Autodesk Inventor part; units mm, degrees
ref_plane "YZ Plane" through (0, 0, 0) normal (1, 0, 0) x (0, 1, 0)
ref_plane "XZ Plane" through (0, 0, 0) normal (0, 1, 0) x (-1, 0, 0)
ref_plane "XY Plane" through (0, 0, 0) normal (0, 0, 1) x (1, 0, 0)
sketch "Sketch1" plane through (0, 0, 0) normal (0, 1, 0) x (-1, 0, 0)
  line L0 (40.1367, 46.4954) -> (-10.6633, 46.4954)
  line L1 (-10.6633, 46.4954) -> (-10.6633, -55.1046)
  line L2 (-10.6633, -55.1046) -> (40.1367, -55.1046)
  line L3 (40.1367, -55.1046) -> (40.1367, 46.4954)
  circle A0 centre (14.7367, -4.3046) radius 12.7
  point P0 (0, 0)
  dimension "d0" = 101.6
  dimension "d1" = 50.8
  dimension "d21" = 25.4
  dimension "d22" = 50.8
extrude "Extrusion1" add sketch "Sketch1" along normal blind 25.4
sketch "Sketch2" plane through (-40.1367, 0, 46.4954) normal (0, 0, 1) x (1, 0, 0)
  line L0 (12.7, 19.8094) -> (36.1, 19.8094)
  line L1 (38.1, 17.8094) -> (38.1, 7.1094)
  line L2 (38.1, 7.1094) -> (12.7, 7.1094)
  line L3 (12.7, 7.1094) -> (12.7, 19.8094)
  line L4 (50.8, 0) -> (50.8, 25.4)
  line L5 (0, 0) -> (0, 25.4)
  arc A0 (38.1, 17.8094) -> (36.1, 19.8094) centre (36.1, 17.8094) ccw
  point P0 (40.1367, 0)
  point P1 (38.1, 19.8094)
  dimension "d5" = 25.4
  dimension "d6" = 12.7
  dimension "d7" = 12.7
  dimension "d8" = 12.7
  dimension "d9" = 12.7
  dimension "d10" = 2
extrude "Extrusion2" cut sketch "Sketch2" against normal up to next
equation "\"d1\" = 0.5 * d0"
equation "\"d21\" = 0.5 * d1"
equation "\"d22\" = 0.5 * d0"
properties part number "Block"
Geometry check sheet. Reference: the model listing, model coordinates, mm. A direction names the side the tool comes from. Give positions to 0.01 mm unless a question says otherwise; leave off trailing zeros. Order: outer loops, then holes, each group sorted by start corner. A loop starts at its lowest first (then second) coordinate and runs counter-clockwise, first axis right, second up.
1. Sectioned sample at C-C (x = -23.5). Record the boundary of the cut face in (y, z).
Completed:
outline: (0, -55.1) - (25.4, -55.1) - (25.4, -13.5) - (0, -13.5) - close; (0, 4.89) - (7.11, 4.89) - (7.11, 46.5) - (0, 46.5) - close; (19.81, 4.89) - (25.4, 4.89) - (25.4, 46.5) - (19.81, 46.5) - close
2. Depth check by flat-ended pin: pin 1 (1 mm diameter, centred on x = -15, z = -14.5, fed in from +Y); pin 2 (2 mm diameter, centred on x = -14.5, y = 12.5, fed in from +Z). Enter the tip coordinate at first touch or a pass-through.
Completed:
pin 1: passes through
pin 2: stops at z = -16.94
3. Sectioned sample at D-D (z = -7.5). Record the boundary of the cut face in (x, y).
Completed:
outline: (-40.14, 0) - (-27.03, 0) - (-27.03, 25.4) - (-40.14, 25.4) - close; (-2.45, 0) - (10.66, 0) - (10.66, 25.4) - (-2.45, 25.4) - close
4. Draft check along Z on faces 1 (the face through (-14, 13, -55.105)), 2 (the face through (-15.1, 6.9, 46.495)), 3 (the face through (-13.1, 12.5, -16.9)), 4 (the face through (-9, 25.4, 8)). Enter one of: pulls with the +Z half, pulls with the -Z half, needs draft (parallel to the pull), parting line crosses it, or undercut.
Completed:
face 1: pulls with the -Z half
face 2: pulls with the +Z half
face 3: undercut
face 4: needs draft
5. Sectioned sample at B-B (y = 9.5). Record the boundary of the cut face in (x, z).
Completed:
outline: (-40.14, -55.1) - (10.66, -55.1) - (10.66, 46.5) - (-2.04, 46.5) - (-2.04, -4.3) arc R12.7 cw to (-27.44, -4.3) - (-27.44, 46.5) - (-40.14, 46.5) - close
6. Access from +Z, -Z, +X, -X, +Y, -Y to the whole of each face (thin tool, end or side, straight path). Record for faces 5 (the face through (10.663, 13, -4)), 6 (the face through (-27.437, 13, 21)).
Completed:
face 5: +Z, -Z, +X, +Y, -Y
face 6: +Z
7. Sectioned sample at A-A (z = 10). Record the boundary of the cut face in (x, y).
Completed:
outline: (-40.14, 0) - (10.66, 0) - (10.66, 25.4) - (-40.14, 25.4) - close; hole (-27.44, 7.11) - (-2.04, 7.11) - (-2.04, 17.81) arc R2 ccw to (-4.04, 19.81) - (-27.44, 19.81) - close
8. Scan lines: line 1 (X direction, y = 10, z = 39); line 2 (Y direction, x = -18, z = 14); line 3 (Z direction, x = -12, y = 17.75). Record each from-to range of solid material in increasing order.
Completed:
line 1: x = -40.14 to -27.44, -2.04 to 10.66
line 2: y = 0 to 7.11, 19.81 to 25.4
line 3: z = -55.1 to -16.71
